from build123d import *

# Parameters (mm, degrees)
SKETCH1_W                 = 12.3
SKETCH1_H                 = 7
BOSS_EXTRUDE1_DEPTH       = 7
SKETCH2_W                 = 11.2
SKETCH2_H                 = 4.6
CUT_EXTRUDE1_DEPTH        = 2.9
SKETCH4_R                 = 2
BOSS_EXTRUDE2_DEPTH       = 6.8
SKETCH5_R                 = 2.7
BOSS_EXTRUDE3_DEPTH       = 35.2
SKETCH6_R                 = 4.3
BOSS_EXTRUDE4_DEPTH       = 4
SKETCH7_W                 = 35.2
SKETCH7_H                 = 1.2
CUT_EXTRUDE2_DEPTH        = 2.9
MIRROR4_COPY_1_SKETCH_W   = 35.2
MIRROR4_COPY_1_SKETCH_H   = 1.2
MIRROR4_COPY_1_DEPTH      = 2.9
CUT_EXTRUDE3_REACH        = 48.762
CUT_EXTRUDE3_END_RADIUS   = 4.3
SKETCH9_W                 = 1.6
SKETCH9_H                 = 2.5
MIRROR6_COPY_1_REACH      = 48.762
MIRROR6_COPY_1_END_RADIUS = 4.3
MIRROR6_COPY_1_SKETCH_W   = 1.6
MIRROR6_COPY_1_SKETCH_H   = 2.5
SKETCH10_W                = 1.4
SKETCH10_H                = 1.2
SKETCH10_W_2              = 1.2
SKETCH10_H_2              = 1.4
BOSS_EXTRUDE5_DEPTH       = 1.2
SKETCH11_R                = 2.7
BOSS_EXTRUDE6_DEPTH       = 1.2
SKETCH12_W                = 1.2
SKETCH12_H                = 1.2
BOSS_EXTRUDE9_DEPTH       = 0.8
FILLET3_R                 = 3.5
SKETCH14_W                = 1
SKETCH14_H                = 12
CUT_EXTRUDE8_DEPTH        = 5


with BuildPart() as part:
    # Sketch1 → Boss-Extrude1 (new body)
    with BuildSketch(Plane(origin=(0, 0, 0), x_dir=(1, 0, 0), z_dir=(0, 1, 0))):
        Rectangle(SKETCH1_W, SKETCH1_H)
    extrude(amount=BOSS_EXTRUDE1_DEPTH)

    # Sketch2 → Cut-Extrude1 (cut)
    with BuildSketch(Plane(origin=(0, 7, 0), x_dir=(1, 0, 0), z_dir=(0, 1, 0))):
        with Locations((0.55, 0)):
            Rectangle(SKETCH2_W, SKETCH2_H)
    cut_extrude1 = extrude(amount=-CUT_EXTRUDE1_DEPTH, mode=Mode.SUBTRACT)

    # Mirror1: Cut-Extrude1 across plane
    add(cut_extrude1.mirror(Plane.ZX.offset(3.5)), mode=Mode.SUBTRACT)

    # Sketch4 → Boss-Extrude2 (add)
    with BuildSketch(Plane.XY.offset(3.5)):
        with Locations(Location((2.45, 3.5, 0), (0, 0, 180))):
            Circle(SKETCH4_R)
    boss_extrude2 = extrude(amount=BOSS_EXTRUDE2_DEPTH)

    # Mirror2: Boss-Extrude2 across plane
    add(boss_extrude2.mirror(Plane.XY))

    # Sketch5 → Boss-Extrude3 (add)
    with BuildSketch(Plane.ZY.offset(6.15)):
        with Locations((0, 3.5)):
            Circle(SKETCH5_R)
    extrude(amount=BOSS_EXTRUDE3_DEPTH)

    # Sketch6 → Boss-Extrude4 (add)
    with BuildSketch(Plane.ZY.offset(41.35)):
        with Locations((0, 3.5)):
            Circle(SKETCH6_R)
    extrude(amount=BOSS_EXTRUDE4_DEPTH)

    # Sketch7 → Cut-Extrude2 (cut)
    with BuildSketch(Plane(origin=(0, 0, 0), x_dir=(-1, 0, 0), z_dir=(0, -1, 0))):
        with Locations((23.75, 1.2)):
            Rectangle(SKETCH7_W, SKETCH7_H)
    cut_extrude2 = extrude(amount=-CUT_EXTRUDE2_DEPTH, mode=Mode.SUBTRACT)

    # Mirror3: Cut-Extrude2 across plane
    add(cut_extrude2.mirror(Plane.ZX.offset(3.5)), mode=Mode.SUBTRACT)

    # Mirror4: Cut-Extrude2 across plane
    add(cut_extrude2.mirror(Plane.XY), mode=Mode.SUBTRACT)

    # Mirror4 copy 1 sketch → Mirror4 copy 1 (cut)
    with BuildSketch(Plane(origin=(0, 7, 0), x_dir=(-1, 0, 0), z_dir=(0, 1, 0))):
        with Locations((23.75, 1.2)):
            Rectangle(MIRROR4_COPY_1_SKETCH_W, MIRROR4_COPY_1_SKETCH_H)
    extrude(amount=-MIRROR4_COPY_1_DEPTH, mode=Mode.SUBTRACT)

    # Cut-Extrude3: up to this cylinder (the profile starts inside it)
    cut_extrude3_end = Plane(origin=(-43.35, 3.5, 0), z_dir=(1, 0, 0)) * Cylinder(CUT_EXTRUDE3_END_RADIUS, 107.124, mode=Mode.PRIVATE)
    # Sketch9 → Cut-Extrude3 (cut, up to the surface)
    with BuildSketch(Plane(origin=(0, 4.1, 0), x_dir=(1, 0, 0), z_dir=(0, 1, 0)), mode=Mode.PRIVATE) as cut_extrude3_sk1:
        with Locations((-43.35, -1.85)):
            Rectangle(SKETCH9_W, SKETCH9_H)
    cut_extrude3_tool1 = extrude(cut_extrude3_sk1.sketch, amount=CUT_EXTRUDE3_REACH, mode=Mode.PRIVATE) & cut_extrude3_end
    cut_extrude3 = cut_extrude3_tool1.solids().sort_by_distance((-43.35, 4.1, 1.85))[0]
    add(cut_extrude3, mode=Mode.SUBTRACT)

    # Mirror5: Cut-Extrude3 across plane
    add(cut_extrude3.mirror(Plane.ZX.offset(3.5)), mode=Mode.SUBTRACT)

    # Mirror6: Cut-Extrude3 across plane
    add(cut_extrude3.mirror(Plane.XY), mode=Mode.SUBTRACT)

    # Mirror6 copy 1: up to this cylinder (the profile starts inside it)
    mirror6_copy_1_end = Plane(origin=(-43.35, 3.5, 0), z_dir=(1, 0, 0)) * Cylinder(MIRROR6_COPY_1_END_RADIUS, 107.124, mode=Mode.PRIVATE)
    # Mirror6 copy 1 sketch → Mirror6 copy 1 (cut, up to the surface)
    with BuildSketch(Plane.XZ.offset(-2.9), mode=Mode.PRIVATE) as mirror6_copy_1_sk1:
        with Locations((-43.35, -1.85)):
            Rectangle(MIRROR6_COPY_1_SKETCH_W, MIRROR6_COPY_1_SKETCH_H)
    mirror6_copy_1_tool1 = extrude(mirror6_copy_1_sk1.sketch, amount=MIRROR6_COPY_1_REACH, mode=Mode.PRIVATE) & mirror6_copy_1_end
    add(mirror6_copy_1_tool1.solids().sort_by_distance((-43.35, 4.1, 1.85))[0], mode=Mode.SUBTRACT)

    # Sketch10 → Boss-Extrude5 (add)
    with BuildSketch(Plane.ZY.offset(45.35)):
        with Locations((1.3, 3.5)):
            Rectangle(SKETCH10_W, SKETCH10_H)
        with Locations((0, 2.2)):
            Rectangle(SKETCH10_W_2, SKETCH10_H_2)
        with Locations((-1.3, 3.5)):
            Rectangle(SKETCH10_W, SKETCH10_H)
        with Locations((0, 4.8)):
            Rectangle(SKETCH10_W_2, SKETCH10_H_2)
        with Locations((0, 3.5)):
            Rectangle(SKETCH10_W_2, SKETCH10_H)
    extrude(amount=BOSS_EXTRUDE5_DEPTH)

    # Sketch11 → Boss-Extrude6 (add)
    with BuildSketch(Plane.ZY.offset(46.55)):
        with Locations((0, 3.5)):
            Circle(SKETCH11_R)
    extrude(amount=BOSS_EXTRUDE6_DEPTH)

    # Sketch12 → Boss-Extrude9 (add)
    with BuildSketch(Plane.ZY.offset(47.75)):
        with BuildLine():
            Line((-2.632489316, 2.9), (-0.6, 2.9))
            Line((-0.6, 2.9), (-0.6, 4.1))
            Line((-0.6, 4.1), (-2.632489316, 4.1))
            ThreePointArc((-2.632489316, 4.1), (-2.683069246, 3.801893066), (-2.7, 3.5))
            ThreePointArc((-2.7, 3.5), (-2.683069246, 3.198106934), (-2.632489316, 2.9))
        make_face()
        with BuildLine():
            Line((-0.6, 4.1), (0.6, 4.1))
            Line((0.6, 4.1), (0.6, 6.132489316))
            ThreePointArc((0.6, 6.132489316), (0.301893066, 6.183069246), (0, 6.2))
            ThreePointArc((0, 6.2), (-0.301893066, 6.183069246), (-0.6, 6.132489316))
            Line((-0.6, 6.132489316), (-0.6, 4.1))
        make_face()
        with BuildLine():
            Line((0.6, 2.9), (2.632489316, 2.9))
            ThreePointArc((2.632489316, 2.9), (2.683069246, 3.198106934), (2.7, 3.5))
            ThreePointArc((2.7, 3.5), (2.683069246, 3.801893066), (2.632489316, 4.1))
            Line((2.632489316, 4.1), (0.6, 4.1))
            Line((0.6, 4.1), (0.6, 2.9))
        make_face()
        with BuildLine():
            Line((0.6, 0.867510684), (0.6, 2.9))
            Line((0.6, 2.9), (-0.6, 2.9))
            Line((-0.6, 2.9), (-0.6, 0.867510684))
            ThreePointArc((-0.6, 0.867510684), (-0.301893067, 0.816930754), (-2e-09, 0.8))
            ThreePointArc((-2e-09, 0.8), (0.301893065, 0.816930754), (0.6, 0.867510684))
        make_face()
        with Locations((0, 3.5)):
            Rectangle(SKETCH12_W, SKETCH12_H)
    extrude(amount=BOSS_EXTRUDE9_DEPTH)

    # Sketch13 → Cut-Revolve6 (revolve, cut)
    with BuildSketch(Plane.XY, mode=Mode.PRIVATE) as cut_revolve6_sk:
        with BuildLine():
            Line((-47.75, 6.2), (-50.26441212, 6.868281128))
            Line((-50.26441212, 6.868281128), (-50.691294746, 5.219710686))
            Line((-50.691294746, 5.219710686), (-49.924832778, 3.5))
            Line((-49.924832778, 3.5), (-48.55, 3.5))
            ThreePointArc((-48.55, 3.5), (-48.380201095, 4.918207732), (-47.75, 6.2))
        make_face()
    revolve(cut_revolve6_sk.sketch.rotate(Axis((-48.75, 3.5, 0), (-1, 0, 0)), 77.160411593), axis=Axis((-48.75, 3.5, 0), (-1, 0, 0)), mode=Mode.SUBTRACT)

    # Fillet3
    fillet3_edges = [part.edges().sort_by_distance(p)[0] for p in [
        (6.15, 0, 2.9),
        (6.15, 7, 2.9),
    ]]
    fillet(fillet3_edges, radius=FILLET3_R - 0.0001)  # a hair under: the kernel refuses the full size

    # Sketch14 → Cut-Extrude8 (cut)
    with BuildSketch(Plane.ZY.offset(45.35)):
        with Locations((-4.5, 3.5)):
            Rectangle(SKETCH14_W, SKETCH14_H)
        with Locations((4.5, 3.5)):
            Rectangle(SKETCH14_W, SKETCH14_H)
    extrude(amount=-CUT_EXTRUDE8_DEPTH, mode=Mode.SUBTRACT)


solid = part.part
Geometry check sheet. Reference: the model listing, model coordinates, mm. A direction names the side the tool comes from. Round coordinates to 2 decimals unless told otherwise and drop trailing zeros. Loops run counter-clockwise (first coordinate to the right, second up) from the corner with the lowest first, then second, coordinate; pieces in that order, holes last. Notation, with made-up numbers: (-16, 16.5) -> (1, 16.5) arc R24 cw to (1, 27.5) -> close; hole circle Ø7 at (-36, -21). An arc over 180 degrees is marked (long way). Answer as a JSON object with one key per item and string values. Group by question number.
Item 1: Cross-section at A-A, the plane x = -30. Record the cut outline in (y, z).
Item 2: Release check for a two-part mould opening along Z. For faces 5 (the face through (-45.9, 3.5, -2)), 6 (the face through (-46, 2.9, -1)), 7 (the face through (-44.15, 6, -2)) record: pulls with the +Z half, pulls with the -Z half, needs draft (parallel to the pull), parting line crosses it, or undercut.
Item 3: Depth check by flat-ended pin: pin 1 Ø1.8 at (x, y) = (-43.5, 1) entering from -Z; pin 2 Ø3 at (x, y) = (-26.5, 4.5) entering from +Z; pin 3 Ø0.8 at (x, z) = (-48, -2) entering from -Y. Enter the tip coordinate at first touch or a pass-through.
Item 4: Thickness scan on line 1 along X through (y, z) = (0.5, -1); line 2 along Z through (x, y) = (-9.5, 2.25); line 3 along Z through (x, y) = (-35, 5.75). Record the ranges inside material, lowest first.
Item 5: Cross-section at B-B, the plane z = 9.25. Record the cut outline in (x, y), plus the area to 3 significant figures.
Item 6: Set-up check for faces 1 (the face through (-44.15, 1, 2)), 2 (the face through (0, 4.1, 0)), 3 (the face through (0, 1, 2.3)), 4 (the face through (-47.75, 2, 1)): record each of +Z, -Z, +X, -X, +Y, -Y from which the full face is reachable in a straight line by a thin tool's end or side.
Item 7: Cross-section at C-C, the plane x = 1.5. Record the cut outline in (y, z), plus the area to 3 significant figures.
Determined:
{
 "1": {"outline": "(0.87, -0.6) -> (2.9, -0.6) -> (2.9, -1.8) -> (1.49, -1.8) arc R2.7 ccw to (5.51, -1.8) -> (4.1, -1.8) -> (4.1, -0.6) -> (6.13, -0.6) arc R2.7 ccw to (6.13, 0.6) -> (4.1, 0.6) -> (4.1, 1.8) -> (5.51, 1.8) arc R2.7 ccw to (1.49, 1.8) -> (2.9, 1.8) -> (2.9, 0.6) -> (0.87, 0.6) arc R2.7 ccw to start"},
 "2": {"face 5": "pulls with the -Z half", "face 6": "needs draft", "face 7": "undercut"},
 "3": {"pin 1": "stops at z = -3.99", "pin 2": "stops at z = 2.7", "pin 3": "stops at y = 1.39"},
 "4": {"line 1": "x = -45.35 to -44.15, -42.55 to -41.35, -6.15 to -5.05", "line 2": "z = -2.39 to -1.8, -0.6 to 0.6, 1.8 to 2.39", "line 3": "z = -0.6 to 0.6"},
 "5": {"outline": "circle Ø4 at (2.45, 3.5)", "area": "12.6 mm²"},
 "6": {"face 1": "-Y", "face 2": "+X, +Y", "face 3": "+X, -Y", "face 4": "+Z, -X, -Y"},
 "7": {"outline": "(0, -3.5) -> (1.74, -3.5) -> (1.74, -10.3) -> (5.26, -10.3) -> (5.26, -3.5) -> (7, -3.5) -> (7, -2.3) -> (4.1, -2.3) -> (4.1, 2.3) -> (7, 2.3) -> (7, 3.5) -> (5.26, 3.5) -> (5.26, 10.3) -> (1.74, 10.3) -> (1.74, 3.5) -> (0, 3.5) -> (0, 2.3) -> (2.9, 2.3) -> (2.9, -2.3) -> (0, -2.3) -> close", "area": "70.2 mm²"}
}
